CAD build for the part. Positions are in the model's coordinates, mm. A direction names the side the tool comes from. Round coordinates to 2 decimals unless told otherwise and drop trailing zeros. Loops run counter-clockwise (first coordinate to the right, second up) from the corner with the lowest first, then second, coordinate; pieces in that order, holes last. Notation, with made-up numbers: (56, -39) -> (64, -39) arc R6 cw to (64, -34) -> close; hole circle Ø3 at (17.25, 67). An arc over 180 degrees is marked (long way). Answer as CSV lines item,"result".
```python
from build123d import *

# Parameters (mm, degrees)
SKETCH1_R           = 1.75
BOSS_EXTRUDE1_DEPTH = 4
SKETCH2_R           = 4
SKETCH2_R_2         = 1.75
BOSS_EXTRUDE2_DEPTH = 3.5


with BuildPart() as part:
    # Sketch1 → Boss-Extrude1 (new body)
    with BuildSketch(Plane.XZ):
        with BuildLine():
            Line((26.669872981, 2.5), (4.330127019, 2.5))
            ThreePointArc((4.330127019, 2.5), (3.348146513, 2.665266452), (2.474358297, 3.142857143))
            ThreePointArc((2.474358297, 3.142857143), (-4, 0), (2.474358297, -3.142857143))
            ThreePointArc((2.474358297, -3.142857143), (3.348146513, -2.665266452), (4.330127019, -2.5))
            Line((4.330127019, -2.5), (26.669872981, -2.5))
            ThreePointArc((26.669872981, -2.5), (27.651853487, -2.665266452), (28.525641703, -3.142857143))
            ThreePointArc((28.525641703, -3.142857143), (35, 0), (28.525641703, 3.142857143))
            ThreePointArc((28.525641703, 3.142857143), (27.651853487, 2.665266452), (26.669872981, 2.5))
        make_face()
        with Locations(Location((31, 0, 0), (0, 0, 90))):
            Circle(SKETCH1_R, mode=Mode.SUBTRACT)
        with Locations(Location((0, 0, 0), (0, 0, 90))):
            Circle(SKETCH1_R, mode=Mode.SUBTRACT)
    extrude(amount=-BOSS_EXTRUDE1_DEPTH)

    # Sketch2 → Boss-Extrude2 (add)
    with BuildSketch(Plane(origin=(0, 4, 0), x_dir=(1, 0, 0), z_dir=(0, 1, 0))):
        with Locations(Location((31, 0, 0), (0, 0, 128.213210702))):
            Circle(SKETCH2_R)
        with Locations(Location((31, 0, 0), (0, 0, 270))):
            Circle(SKETCH2_R_2, mode=Mode.SUBTRACT)
    extrude(amount=BOSS_EXTRUDE2_DEPTH)


solid = part.part
```
Q1. Slice it at D-D, the plane y = 5.5. Give the cut face in (x, z), and give its area (3 significant figures).
Results:
outline,"circle Ø8 at (31, 0); hole circle Ø3.5 at (31, 0)"
area,"40.6 mm2"
Q2. Drop flat-ended pins along their axis: pin 1 Ø2 at (x, y) = (10, 1.5) entering from -Z; pin 2 Ø1 at (x, y) = (28.5, 4.5) entering from -Z; pin 3 Ø1.5 at (y, z) = (1.5, -2) entering from -X; pin 4 Ø4.5 at (x, z) = (0, 0) entering from -Y. Give the stop position or say it passes through.
Results:
pin 1,"z = -2.5"
pin 2,"z = -3.46"
pin 3,"x = -3.8"
pin 4,"y = 0"
Q3. Two-plate mould, pull along X, no slides. Class faces 4 (the flat face through (15, 0, 0)), 5 (the cylindrical face through (3.33, 1.97, -2.67)): pulls with the +X half, pulls with the -X half, needs draft (parallel to the pull), parting line crosses it, or undercut.
Results:
face 4,"needs draft"
face 5,"undercut"
Q4. Probe L1, parallel to Z at x = 31, y = 5.85; L2, parallel to X at y = 6.5, z = 0; L3, parallel to Y at x = 21, z = -0.5. List the from-to ranges inside material, lowest first. Write a range as [from, to].
Results:
L1,"[-4, -1.75], [1.75, 4]"
L2,"[27, 29.25], [32.75, 35]"
L3,"[0, 4]"
Q5. Slice it at C-C, the plane y = 1. Give the cut face in (x, z), and give its area (3 significant figures).
Results:
outline,"(2.47, -3.14) arc R3 cw to (4.33, -2.5) -> (26.67, -2.5) arc R3 cw to (28.53, -3.14) arc R4 ccw (long way) to (28.53, 3.14) arc R3 cw to (26.67, 2.5) -> (4.33, 2.5) arc R3 cw to (2.47, 3.14) arc R4 ccw (long way) to start; hole circle Ø3.5 at (0, 0); hole circle Ø3.5 at (31, 0)"
area,"200 mm2"
Q6. Tool access for faces 1 (the cylindrical face through (-4, 2, 0)), 2 (the cylindrical face through (3.36, 1.97, 2.66)), 3 (the flat face through (15, 2, -2.5)): list every direction of +Z, -Z, +X, -X, +Y, -Y with a clear straight run to the whole face (end or side of a thin tool).
Results:
face 1,"+Y, -Y"
face 2,"+Z, +Y, -Y"
face 3,"-Z, +Y, -Y"
Q7. Slice it at A-A, the plane z = 0. Give the cut face in (x, y), and give its area (3 significant figures).
Results:
outline,"(-4, 0) -> (-1.75, 0) -> (-1.75, 4) -> (-4, 4) -> close; (1.75, 0) -> (29.25, 0) -> (29.25, 7.5) -> (27, 7.5) -> (27, 4) -> (1.75, 4) -> close; (32.75, 0) -> (35, 0) -> (35, 7.5) -> (32.75, 7.5) -> close"
area,"144 mm2"
Q8. Slice it at B-B, the plane x = 31. Give the cut face in (y, z), and give its area (4 significant figures).
Results:
outline,"(0, -4) -> (7.5, -4) -> (7.5, -1.75) -> (0, -1.75) -> close; (0, 1.75) -> (7.5, 1.75) -> (7.5, 4) -> (0, 4) -> close"
area,"33.75 mm2"
